For this review, take the finished solid that the model builds, in its own axes (mm). A direction names the side the tool comes from. Coordinates: 2 decimals unless noted, no trailing zeros. Order: outer loops, then holes, each group sorted by start corner. A loop starts at its lowest first (then second) coordinate and runs counter-clockwise, first axis right, second up. Notation, with made-up numbers: (45, 23.5) -> (61, 23.5) arc R27 ccw to (61, 58.5) -> close; hole circle Ø4 at (-21, 22.5). An arc over 180 degrees is marked (long way). Return JSON: item names as keys, results as strings. Group by question number.
Item 1: Take a section at C-C (y = 7). Write out the cut boundary in (x, z).
Item 2: Machinability: for faces 1 (the flat face through (0.2, -2, -6.5)), 2 (the cylindrical face through (-0.67, 14.86, -58.383)), 3 (the cylindrical face through (0.66, -13.479, 14.985)), which of the approach directions +Z, -Z, +X, -X, +Y, -Y give a long, thin tool a straight path to every point of the face, cutting with its end or side? Answer none if there is none.
Item 3: For line 1 along Y through (x, z) = (-22, -12); line 2 along Z through (x, y) = (-0.5, 23.5); line 3 along X through (y, z) = (-5, -5), list the stretches that pass through material, from the lowest coordinate up.
Item 4: Insertion check: pin 1 (6 mm diameter, centred on x = -26, z = 24, fed in from +Y); pin 2 (4 mm diameter, centred on x = 55, z = -44.5, fed in from -Y); pin 3 (10 mm diameter, centred on x = -8.5, y = -7.5, fed in from -Z). Each pin has a flat end and moves straight along its axis. Give the tip position at first contact, or say it passes through.
Item 5: Take a section at D-D (y = -7). Write out the cut boundary in (x, z).
Item 6: Take a section at B-B (x = -13). Write out the cut boundary in (y, z), then the cut area to 3 significant figures.
Item 7: Draft analysis for pull direction X (two halves, no side actions). For faces 4 (the cylindrical face through (-61.71, 14.86, -0.38)), 5 (the flat face through (75, 2, 1)), 6 (the cylindrical face through (1.802, -6.93, -5.723)), state which applies: +X half, -X half, draft (parallel to the pull), parting line (faces both ways), or undercut.
Item 8: Take a section at A-A (z = 0). Write out the cut boundary in (x, y).
```python
from build123d import *

# Parameters (mm, degrees)
SKETCH1_W           = 150
SKETCH1_H           = 150
BOSS_EXTRUDE1_DEPTH = 5
SKETCH2_R           = 1.75
BOSS_EXTRUDE2_DEPTH = 20
SKETCH3_R           = 15
BOSS_EXTRUDE4_DEPTH = 2
SKETCH5_R           = 6
BOSS_EXTRUDE5_DEPTH = 10
SKETCH6_R           = 15
BOSS_EXTRUDE6_DEPTH = 3


with BuildPart() as part:
    # Sketch1 → Boss-Extrude1 (new body)
    with BuildSketch(Plane(origin=(0, 0, 0), x_dir=(1, 0, 0), z_dir=(0, 1, 0))):
        Rectangle(SKETCH1_W, SKETCH1_H)
    extrude(amount=BOSS_EXTRUDE1_DEPTH)

    # Sketch2 → Boss-Extrude2 (add)
    with BuildSketch(Plane(origin=(0, 5, 0), x_dir=(1, 0, 0), z_dir=(0, 1, 0))):
        with Locations(Location((-60, 0, 0), (0, 0, 270))):
            Circle(SKETCH2_R)
        with Locations(Location((0, 60, 0), (0, 0, 270))):
            Circle(SKETCH2_R)
        with Locations(Location((60, 0, 0), (0, 0, 270))):
            Circle(SKETCH2_R)
        with Locations(Location((0, -60, 0), (0, 0, 270))):
            Circle(SKETCH2_R)
    extrude(amount=BOSS_EXTRUDE2_DEPTH)

    # Sketch3 → Boss-Extrude4 (add)
    with BuildSketch(Plane.XZ):
        with Locations(Location((0, 0, 0), (0, 0, 270))):
            Circle(SKETCH3_R)
    extrude(amount=BOSS_EXTRUDE4_DEPTH)

    # Sketch5 → Boss-Extrude5 (add)
    with BuildSketch(Plane.XZ.offset(2)):
        with Locations(Location((0, 0, 0), (0, 0, 270))):
            Circle(SKETCH5_R)
    extrude(amount=BOSS_EXTRUDE5_DEPTH)

    # Sketch6 → Boss-Extrude6 (add)
    with BuildSketch(Plane.XZ.offset(12)):
        with Locations(Location((0, 0, 0), (0, 0, 270))):
            Circle(SKETCH6_R)
    extrude(amount=BOSS_EXTRUDE6_DEPTH)


solid = part.part
```
Findings below:
{
 "1": {"outline": "circle Ø3.5 at (-60, 0); circle Ø3.5 at (0, -60); circle Ø3.5 at (0, 60); circle Ø3.5 at (60, 0)"},
 "2": {"face 1": "none", "face 2": "+Y", "face 3": "-Y"},
 "3": {"line 1": "y = 0 to 5", "line 2": "z = -61.68 to -58.32, 58.32 to 61.68", "line 3": "x = -3.32 to 3.32"},
 "4": {"pin 1": "stops at y = 5", "pin 2": "stops at y = 0", "pin 3": "stops at z = -13.6"},
 "5": {"outline": "circle Ø12 at (0, 0)"},
 "6": {"outline": "(-15, -7.48) -> (-12, -7.48) -> (-12, 7.48) -> (-15, 7.48) -> close; (-2, -7.48) -> (0, -7.48) -> (0, -75) -> (5, -75) -> (5, 75) -> (0, 75) -> (0, 7.48) -> (-2, 7.48) -> close", "area": "825 mm2"},
 "7": {"face 4": "undercut", "face 5": "+X half", "face 6": "parting line"},
 "8": {"outline": "(-75, 0) -> (-15, 0) -> (-15, -2) -> (-6, -2) -> (-6, -12) -> (-15, -12) -> (-15, -15) -> (15, -15) -> (15, -12) -> (6, -12) -> (6, -2) -> (15, -2) -> (15, 0) -> (75, 0) -> (75, 5) -> (61.75, 5) -> (61.75, 25) -> (58.25, 25) -> (58.25, 5) -> (-58.25, 5) -> (-58.25, 25) -> (-61.75, 25) -> (-61.75, 5) -> (-75, 5) -> close"}
}
